Can you work these out from the model? Positions are in its coordinate system, mm. A direction names the side the tool comes from. Round coordinates to 2 decimals unless told otherwise and drop trailing zeros. Loops run counter-clockwise (first coordinate to the right, second up) from the corner with the lowest first, then second, coordinate; pieces in that order, holes last. Notation, with made-up numbers: (-26.5, 76) -> (5.5, 76) arc R25 ccw to (5.5, 100) -> close; hole circle Ø8 at (29, 38.5). An arc over 180 degrees is marked (long way). Use a Markdown table: item, result.
from build123d import *

# Parameters (mm, degrees)
SKETCH_1_W               = 15.2
SKETCH_1_H               = 15.2
EXTRUDE_1_DEPTH          = 20
SKETCH_2_W               = 25.2
SKETCH_2_H               = 25.2
SKETCH_2_W_2             = 15.2
SKETCH_2_H_2             = 15.2
EXTRUDE_2_DEPTH          = 15
SKETCH_3_W               = 15.2
SKETCH_3_H               = 15.2
CUT_EXTRUDE_1_DEPTH      = 80
SKETCH_4_R               = 1.6
CUT_EXTRUDE_2_DEPTH      = 83.635888087
FILLET_1_R               = 5
SKETCH_5_W               = 15.2
SKETCH_5_H               = 15.2
CUT_EXTRUDE_3_DEPTH      = 83.635888087
CUT_EXTRUDE_5_DEPTH      = 72.228786316
CUT_EXTRUDE_5_DEPTH_BACK = 72.228786316
SKETCH_7_R               = 1.6
SKETCH_8_W               = 47
SKETCH_8_H               = 5
EXTRUDE_3_DEPTH          = 8
CUT_EXTRUDE_6_REACH      = 84.636
SKETCH_9_R               = 21.25
SKETCH_9_R_2             = 1.4
FILLET_2_R               = 5


with BuildPart() as part:
    # 草图1 → 凸台-拉伸1 (new body)
    with BuildSketch(Plane(origin=(0, 0, 0), x_dir=(1, 0, 0), z_dir=(0, 1, 0))):
        Polygon((-37.5, 12.5), (-12.6, 12.5), (-12.6, 27.7), (12.6, 27.7), (12.6, 12.5), (30, 12.5), (30, -13.5), (-62.5, -13.5), (-62.5, 22.5), (-37.5, 22.5), align=None)
        with Locations((0, 15.1)):
            Rectangle(SKETCH_1_W, SKETCH_1_H, mode=Mode.SUBTRACT)
    extrude(amount=EXTRUDE_1_DEPTH)

    # 草图2 → 凸台-拉伸2 (add)
    with BuildSketch(Plane(origin=(0, 20, 0), x_dir=(1, 0, 0), z_dir=(0, 1, 0))):
        with Locations((0, 15.1)):
            Rectangle(SKETCH_2_W, SKETCH_2_H)
        with Locations((0, 15.1)):
            Rectangle(SKETCH_2_W_2, SKETCH_2_H_2, mode=Mode.SUBTRACT)
    extrude(amount=EXTRUDE_2_DEPTH)

    # 草图3 → 切除-拉伸1 (cut)
    with BuildSketch(Plane(origin=(30, 0, 0), x_dir=(0, 0, -1), z_dir=(1, 0, 0))):
        with Locations((0, 7.6)):
            Rectangle(SKETCH_3_W, SKETCH_3_H)
    extrude(amount=-CUT_EXTRUDE_1_DEPTH, mode=Mode.SUBTRACT)

    # 草图4 → 切除-拉伸2 (cut, through all)
    with BuildSketch(Plane.XY.offset(13.5)):
        with Locations((0, 7.5)):
            Circle(SKETCH_4_R)
        with Locations((25, 7.5)):
            Circle(SKETCH_4_R)
        with Locations((-20, 7.5)):
            Circle(SKETCH_4_R)
        with Locations((0, 27.5)):
            Circle(SKETCH_4_R)
        with Locations((-30, 7.5)):
            Circle(SKETCH_4_R)
    extrude(amount=-CUT_EXTRUDE_2_DEPTH, mode=Mode.SUBTRACT)

    # 圆角1
    fillet_1_edges = [part.edges().sort_by_distance(p)[0] for p in [
        (-37.5, 10, -12.5),
        (-12.6, 10, -12.5),
        (12.6, 10, -12.5),
        (-12.6, 20, -7.5),
        (0, 20, -2.5),
        (12.6, 20, -7.5),
    ]]
    fillet(fillet_1_edges, radius=FILLET_1_R)

    # 草图5 → 切除-拉伸3 (cut, through all)
    with BuildSketch(Plane.XY.offset(13.5)):
        with Locations((-50, 7.6)):
            Rectangle(SKETCH_5_W, SKETCH_5_H)
    extrude(amount=-CUT_EXTRUDE_3_DEPTH, mode=Mode.SUBTRACT)

    # 草图7 → 切除-拉伸5 (cut, two sides: drawn at the far end of the back side and taken through both)
    with BuildSketch(Plane(origin=(0, 20, 0), x_dir=(1, 0, 0), z_dir=(0, 1, 0)).offset(-CUT_EXTRUDE_5_DEPTH_BACK)):
        with Locations(Location((-50, 0, 0), (0, 0, 270))):
            Circle(SKETCH_7_R)
        with Locations(Location((-30, 0, 0), (0, 0, 270))):
            Circle(SKETCH_7_R)
        with Locations(Location((18, 0, 0), (0, 0, 270))):
            Circle(SKETCH_7_R)
        with Locations(Location((-50, 17.5, 0), (0, 0, 270))):
            Circle(SKETCH_7_R)
    extrude(amount=CUT_EXTRUDE_5_DEPTH + CUT_EXTRUDE_5_DEPTH_BACK, mode=Mode.SUBTRACT)

    # 草图8 → 凸台-拉伸3 (add)
    with BuildSketch(Plane(origin=(0, 20, 0), x_dir=(1, 0, 0), z_dir=(0, 1, 0))):
        with Locations((-39, -11)):
            Rectangle(SKETCH_8_W, SKETCH_8_H)
    extrude(amount=EXTRUDE_3_DEPTH)

    # 草图9 → 切除-拉伸6 (cut, up to next)
    with BuildSketch(Plane.XY.offset(13.5), mode=Mode.PRIVATE) as cut_extrude_6_sk1:
        with Locations((-37.5, 47.5)):
            Circle(SKETCH_9_R)
    cut_extrude_6_tool1 = extrude(cut_extrude_6_sk1.sketch, amount=-CUT_EXTRUDE_6_REACH, mode=Mode.PRIVATE) & part.part
    # 草图9 → 切除-拉伸6 (cut, up to next)
    with BuildSketch(Plane.XY.offset(13.5), mode=Mode.PRIVATE) as cut_extrude_6_sk2:
        with Locations((-52.5, 23)):
            Circle(SKETCH_9_R_2)
    cut_extrude_6_tool2 = extrude(cut_extrude_6_sk2.sketch, amount=-CUT_EXTRUDE_6_REACH, mode=Mode.PRIVATE) & part.part
    # 草图9 → 切除-拉伸6 (cut, up to next)
    with BuildSketch(Plane.XY.offset(13.5), mode=Mode.PRIVATE) as cut_extrude_6_sk3:
        with Locations((-22.5, 23)):
            Circle(SKETCH_9_R_2)
    cut_extrude_6_tool3 = extrude(cut_extrude_6_sk3.sketch, amount=-CUT_EXTRUDE_6_REACH, mode=Mode.PRIVATE) & part.part
    add(cut_extrude_6_tool1.solids().sort_by_distance((-37.5, 47.5, 13.5))[0], mode=Mode.SUBTRACT)
    add(cut_extrude_6_tool2.solids().sort_by_distance((-52.5, 23, 13.5))[0], mode=Mode.SUBTRACT)
    add(cut_extrude_6_tool3.solids().sort_by_distance((-22.5, 23, 13.5))[0], mode=Mode.SUBTRACT)

    # 圆角2
    # the kernel refuses this fillet: 5 mm, written as the material it adds along each edge
    with BuildSketch(Plane(origin=(-15.5, 20, 13.5), x_dir=(1, 0, 0), z_dir=(0, 0, -1))) as fillet_2_piece_1:
        with BuildLine():
            CenterArc((FILLET_2_R, -FILLET_2_R), FILLET_2_R, 90, 90)
            Line((0, -FILLET_2_R), (0, 0))
            Line((0, 0), (FILLET_2_R, 0))
        make_face()
    extrude(amount=5)
    with BuildSketch(Plane(origin=(-15.5, 20, 8.5), x_dir=(0, 0, -1), z_dir=(-1, 0, 0))) as fillet_2_piece_2_section:
        with BuildLine():
            CenterArc((FILLET_2_R, -FILLET_2_R), FILLET_2_R, 90, 90)
            Line((0, -FILLET_2_R), (0, 0))
            Line((0, 0), (FILLET_2_R, 0))
        make_face()
    fillet_2_piece_2 = extrude(amount=47, mode=Mode.PRIVATE)
    fillet_2_piece_2 = fillet_2_piece_2 - Plane(origin=(-22.5, 23, 7.347121569), x_dir=(1, 0, 0), z_dir=(0, 0, 1)) * Cylinder(1.4, 114, mode=Mode.PRIVATE)
    fillet_2_piece_2 = fillet_2_piece_2 - Plane(origin=(-52.5, 23, 7.347121569), x_dir=(1, 0, 0), z_dir=(0, 0, 1)) * Cylinder(1.4, 114, mode=Mode.PRIVATE)
    add(fillet_2_piece_2)
    with BuildSketch(Plane(origin=(-3, 20, 8.5), x_dir=(0, 0, -1), z_dir=(-1, 0, 0))) as fillet_2_piece_3a_section:
        with BuildLine():
            CenterArc((FILLET_2_R, -FILLET_2_R), FILLET_2_R, 90, 90)
            Line((0, -FILLET_2_R), (0, 0))
            Line((0, 0), (FILLET_2_R, 0))
        make_face()
    fillet_2_piece_3a = extrude(amount=59.5, mode=Mode.PRIVATE)
    fillet_2_piece_3a = split(fillet_2_piece_3a, bisect_by=Plane(origin=(-15.5, 21.131975571, 7.368024429), z_dir=(1, 0, 0)), keep=Keep.TOP, mode=Mode.PRIVATE)
    with BuildSketch(Plane(origin=(-15.5, 20, 13.5), x_dir=(1, 0, 0), z_dir=(0, 0, -1))) as fillet_2_piece_3b_section:
        with BuildLine():
            CenterArc((FILLET_2_R, -FILLET_2_R), FILLET_2_R, 90, 90)
            Line((0, -FILLET_2_R), (0, 0))
            Line((0, 0), (FILLET_2_R, 0))
        make_face()
    fillet_2_piece_3b = extrude(amount=17.5, mode=Mode.PRIVATE)
    fillet_2_piece_3b = split(fillet_2_piece_3b, bisect_by=Plane(origin=(-14.368024429, 21.131975571, 8.5), z_dir=(0, 0, -1)), keep=Keep.TOP, mode=Mode.PRIVATE)
    fillet_2_piece_3 = fillet_2_piece_3a & fillet_2_piece_3b
    add(fillet_2_piece_3)
    # the kernel refuses this fillet: 5 mm, written as the material it takes off along each edge
    with BuildSketch(Plane(origin=(-29.055327123, 28, 6.051586161), x_dir=(-0.9256891824228564, -0.378284995136344, 0), z_dir=(0, 0, 1))) as fillet_2_2_piece_1:
        with BuildLine():
            CenterArc((0.984836894, 4.998925199), FILLET_2_R, 247.772508302, 21.039469781)
            Line((-0.906588082, 0.370479287), (0, 0))
            ThreePointArc((0, 0), (0.440584926, 0.004567905), (0.881169852, 0))
        make_face()
    extrude(amount=9.896827677, mode=Mode.SUBTRACT)
    with BuildSketch(Plane(origin=(-45.944672877, 28, 6.051586161), x_dir=(-1, 0, 0), z_dir=(0, 0, 1))) as fillet_2_2_piece_2:
        with BuildLine():
            CenterArc((0.979365535, 5), FILLET_2_R, 248.960530219, 21.039469781)
            ThreePointArc((-0.8156894, 0.333333333), (-0.40611673, 0.170895126), (0, 0))
            Line((0, 0), (0.979365535, 0))
        make_face()
    extrude(amount=9.896827677, mode=Mode.SUBTRACT)


solid = part.part
1. I want a section at B-B (y = 10). Please give me the cut outline in (x, z).
Answer sheet:
| item | result |
|---|---|
| outline | (-62.5, -22.5) -> (-57.6, -22.5) -> (-57.6, 13.5) -> (-62.5, 13.5) -> close; (-42.4, -22.5) -> (-37.5, -22.5) -> (-37.5, -17.5) arc R5 cw to (-32.5, -12.5) -> (-17.6, -12.5) arc R5 cw to (-12.6, -17.5) -> (-12.6, -27.7) -> (12.6, -27.7) -> (12.6, -17.5) arc R5 cw to (17.6, -12.5) -> (30, -12.5) -> (30, -7.6) -> (7.6, -7.6) -> (7.6, -22.7) -> (-7.6, -22.7) -> (-7.6, -7.6) -> (-42.4, -7.6) -> close; (-42.4, 7.6) -> (30, 7.6) -> (30, 13.5) -> (-42.4, 13.5) -> close |
2. If we mould it in two halves opening along Y, with no side actions, what happens to faces 4 (the cylindrical face through (-31.27, 6.53, -10.02)), 5 (the cylindrical face through (-45.999, 27.914, 10.965)), 6 (the flat face through (-62.5, 11, -5))? For each: +Y half, -Y half, draft (parallel to the pull), parting line (faces both ways), or undercut.
Answer sheet:
| item | result |
|---|---|
| face 4 | undercut |
| face 5 | +Y half |
| face 6 | draft |
3. I need wall thicknesses on line 1 (X direction, y = 3, z = -18); line 2 (X direction, y = 10, z = -11.5); line 3 (X direction, y = 18.9, z = 0). Which ranges of each line are inside material? Lowest first, please.
Answer sheet:
| item | result |
|---|---|
| line 1 | x = -62.5 to -57.6, -42.4 to -37.5, -12.6 to -7.6, 7.6 to 12.6 |
| line 2 | x = -62.5 to -57.6, -42.4 to -7.6, 7.6 to 30 |
| line 3 | x = -62.5 to -51.6, -48.4 to -31.6, -28.4 to 16.4, 19.6 to 30 |
4. I want a section at D-D (z = 0). Please give me the cut outline in (x, y).
Answer sheet:
| item | result |
|---|---|
| outline | (-62.5, 0) -> (-57.6, 0) -> (-57.6, 15.2) -> (-51.6, 15.2) -> (-51.6, 20) -> (-62.5, 20) -> close; (-48.4, 15.2) -> (-31.6, 15.2) -> (-31.6, 20) -> (-48.4, 20) -> close; (-28.4, 15.2) -> (16.4, 15.2) -> (16.4, 20.15) arc R5 cw to (15.1, 20.67) -> (-15.1, 20.67) arc R5 cw to (-17.6, 20) -> (-28.4, 20) -> close; (19.6, 15.2) -> (30, 15.2) -> (30, 20) -> (19.6, 20) -> close |
5. Which directions (+Z, -Z, +X, -X, +Y, -Y) give clear straight access to the entire face, cutting with the end or side of a thin tool? Please do faces 1 (the flat face through (-7.6, 17, -15)), 2 (the flat face through (-25, 7, -7.6)), 3 (the flat face through (-12.6, 21, -18)).
Answer sheet:
| item | result |
|---|---|
| face 1 | +Y, -Y |
| face 2 | +X, -Y |
| face 3 | -Z, +Y |
6. I want a section at C-C (x = -50). Please give me the cut outline in (y, z).
Answer sheet:
| item | result |
|---|---|
| outline | (15.2, -22.5) -> (20, -22.5) -> (20, -19.1) -> (15.2, -19.1) -> close; (15.2, -15.9) -> (20, -15.9) -> (20, -1.6) -> (15.2, -1.6) -> close; (15.2, 1.6) -> (20, 1.6) -> (20, 3.5) arc R5 cw to (25, 8.5) -> (28, 8.5) -> (28, 13.5) -> (15.2, 13.5) -> close |
7. I want a section at A-A (x = 6.5). Please give me the cut outline in (y, z).
Answer sheet:
| item | result |
|---|---|
| outline | (0, -27.7) -> (35, -27.7) -> (35, -22.7) -> (0, -22.7) -> close; (0, 7.6) -> (15.2, 7.6) -> (15.2, -7.5) -> (35, -7.5) -> (35, -2.5) -> (25, -2.5) arc R5 cw to (20, 2.5) -> (20, 13.5) -> (0, 13.5) -> close |
8. Will these pins go through, and if not, where does the flat tip stop? pin 1 Ø1.5 at (x, z) = (8.5, -11.5) entering from -Y; pin 2 Ø6 at (x, y) = (-44.5, 8.5) entering from -Z; pin 3 Ø3.5 at (x, y) = (-30, 7.5) entering from -Z; pin 4 Ø3.5 at (y, z) = (26, 10.5) entering from +X.
Answer sheet:
| item | result |
|---|---|
| pin 1 | stops at y = 0 |
| pin 2 | stops at z = -22.5 |
| pin 3 | stops at z = -12.5 |
| pin 4 | stops at x = -15.44 |
